Geometry check sheet. Reference: the model listing, model coordinates, mm. Face numbers are marked on the shaded views. Round coordinates to 2 decimals unless told otherwise and drop trailing zeros. Order: outer loops, then holes, each group sorted by start corner. A loop starts at its lowest first (then second) coordinate and runs counter-clockwise, first axis right, second up. Notation, with made-up numbers: (20, 21) -> (78, 21) arc R30 cw to (78, 47) -> close; hole circle Ø10 at (66, -19.5). An arc over 180 degrees is marked (long way). Use a Markdown table: item, result. Add a question column.
Item 1: Material ranges on probe 1 along X at (y, z) = (2.1, 1.25); probe 2 along Z at (x, y) = (-0.5, 0.3); probe 3 along Z at (x, y) = (0, 1.1), recorded low to high. Write a range as [from, to].
Item 2: Sectioned sample at B-B, the plane x = 3.5. Record the cut outline in (y, z).
Item 3: Mould release check, pull along Z, two halves, no side actions. Record for the marked faces 1, 2, 3 and 4: pulls with the +Z half, pulls with the -Z half, needs draft (parallel to the pull), parting line crosses it, or undercut.
Item 4: Sectioned sample at A-A, the plane z = 3. Record the cut outline in (x, y), and give its area (3 significant figures).
from build123d import *

# Parameters (mm, degrees)
SKETCH2_R           = 2.2
BOSS_EXTRUDE1_DEPTH = 3
CHAMFER1_SIZE       = 0.5
THREAD1_PITCH       = 0.7


with BuildPart() as part:
    # Sketch2 → Boss-Extrude1 (new body)
    with BuildSketch(Plane(origin=(0, 0, 0), x_dir=(1, 0, 0), z_dir=(0, 1, 0))):
        Polygon((4.618802154, 0), (2.309401077, 4), (-2.309401077, 4), (-4.618802154, 0), (-2.309401077, -4), (2.309401077, -4), align=None)
        with Locations(Location((0, 0, 0), (0, 0, 270))):
            Circle(SKETCH2_R, mode=Mode.SUBTRACT)
    extrude(amount=BOSS_EXTRUDE1_DEPTH)

    # Chamfer1
    chamfer1_edges = [part.edges().sort_by_distance(p)[0] for p in [
        (0, 0, -2.2),
        (0, 3, -2.2),
    ]]
    chamfer(chamfer1_edges, length=CHAMFER1_SIZE)

    # Thread1: the profile of Thread Profile1 profile screwed along a right-hand helix of 5.714286 turns, 6 arcs to a turn; built about Z, then put on its axis
    thread1_z = Axis((0, 0, 0), (0, 0, 1))
    thread1_corners = [(2.1997, 0, -0.000173205), (2.578886113, 0, 0.218749999), (2.578886113, 0, 0.306249999), (2.1997, 0, 0.525173203)]
    with BuildLine(mode=Mode.PRIVATE) as thread1_profile:
        Line(thread1_corners[0], thread1_corners[1])
        Line(thread1_corners[1], thread1_corners[2])
        Line(thread1_corners[2], thread1_corners[3])
        Line(thread1_corners[3], thread1_corners[0])
    thread1_cap = Face(thread1_profile.wire())
    thread1_turn_angles = [0, 30, 60, 90, 120, 150, 180, 210, 240, 270, 300, 330, 360]
    thread1_turn_weights = [1, 0.8660254037844387, 1, 0.8660254037844387, 1, 0.8660254037844387, 1, 0.8660254037844387, 1, 0.8660254037844387, 1, 0.8660254037844387, 1]
    thread1_turn_rails = [Edge.make_bspline([Vector(p[0], p[1], 0).rotate(thread1_z, thread1_turn_angles[k]) / thread1_turn_weights[k] + Vector(0, 0, p[2] + THREAD1_PITCH * thread1_turn_angles[k] / 360) for k in range(13)], [0, 0, 0, 1, 1, 2, 2, 3, 3, 4, 4, 5, 5, 6, 6, 6], 2, thread1_turn_weights) for p in thread1_corners]
    thread1_turn_sides = [Face.make_surface_from_curves(thread1_turn_rails[p[0]], thread1_turn_rails[p[1]]) for p in [(0, 1), (1, 2), (2, 3), (3, 0)]]
    thread1_last_angles = [1800, 1830, 1860, 1890, 1920, 1950, 1980, 2010, 2040, 2048.571428571, 2057.142857143]
    thread1_last_weights = [1, 0.8660254037844387, 1, 0.8660254037844387, 1, 0.8660254037844387, 1, 0.8660254037844387, 1, 0.9888308262251283, 1]
    thread1_last_rails = [Edge.make_bspline([Vector(p[0], p[1], 0).rotate(thread1_z, thread1_last_angles[k]) / thread1_last_weights[k] + Vector(0, 0, p[2] + THREAD1_PITCH * thread1_last_angles[k] / 360) for k in range(11)], [0, 0, 0, 1, 1, 2, 2, 3, 3, 4, 4, 5, 5, 5], 2, thread1_last_weights) for p in thread1_corners]
    thread1_last_sides = [Face.make_surface_from_curves(thread1_last_rails[p[0]], thread1_last_rails[p[1]]) for p in [(0, 1), (1, 2), (2, 3), (3, 0)]]
    thread1 = Plane(origin=(0, 0.5, 0), x_dir=(1, 0, 0), z_dir=(0, 1, 0)) * Solid(Shell([*[p.moved(Location((0, 0, THREAD1_PITCH * i))) for i in range(5) for p in thread1_turn_sides], *thread1_last_sides, thread1_cap, thread1_cap.rotate(thread1_z, 2057.142857143).moved(Location((0, 0, THREAD1_PITCH * 2057.142857143 / 360)))]))
    add(thread1, mode=Mode.SUBTRACT)


solid = part.part
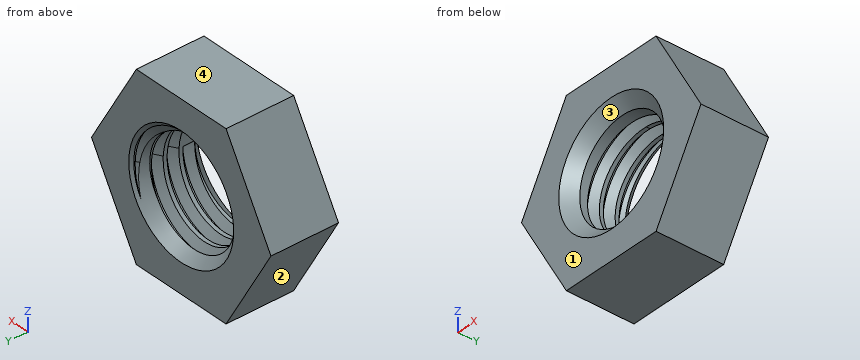
Found:
| question | item | result |
|---|---|---|
| 1 | probe 1 | x = [-3.9, -1.89], [2.26, 3.9] |
| 1 | probe 2 | z = [-4, -2.35], [2.35, 4] |
| 1 | probe 3 | z = [-4, -2.37], [2.33, 4] |
| 2 | outline | (0, -1.94) -> (3, -1.94) -> (3, 1.94) -> (0, 1.94) -> close |
| 3 | face 1 | needs draft |
| 3 | face 2 | pulls with the -Z half |
| 3 | face 3 | undercut |
| 3 | face 4 | pulls with the +Z half |
| 4 | outline | (-2.89, 0) -> (2.89, 0) -> (2.89, 3) -> (-2.89, 3) -> close |
| 4 | area | 17.3 mm2 |
